from build123d import *

# Parameters (mm, degrees)
SKETCH1_W           = 57.912
SKETCH1_H           = 70.104
SKETCH1_R           = 4.25
SKETCH1_R_2         = 6.35
BOSS_EXTRUDE1_DEPTH = 1.5494
FILLET1_R           = 7.62


with BuildPart() as part:
    # Sketch1 → Boss-Extrude1 (new body)
    with BuildSketch(Plane(origin=(0, 0, 0), x_dir=(0, 0, -1), z_dir=(1, 0, 0))):
        Rectangle(SKETCH1_W, SKETCH1_H)
        with Locations((-20.447, 26.543)):
            Circle(SKETCH1_R, mode=Mode.SUBTRACT)
        with Locations((20.447, 26.543)):
            Circle(SKETCH1_R, mode=Mode.SUBTRACT)
        with Locations((20.447, -26.543)):
            Circle(SKETCH1_R, mode=Mode.SUBTRACT)
        with Locations((-20.447, -26.543)):
            Circle(SKETCH1_R, mode=Mode.SUBTRACT)
        Circle(SKETCH1_R_2, mode=Mode.SUBTRACT)
    extrude(amount=BOSS_EXTRUDE1_DEPTH)

    # Fillet1
    fillet1_edges = [part.edges().sort_by_distance(p)[0] for p in [
        (0.7747, -35.052, -28.956),
        (0.7747, -35.052, 28.956),
        (0.7747, 35.052, 28.956),
        (0.7747, 35.052, -28.956),
    ]]
    fillet(fillet1_edges, radius=FILLET1_R)


solid = part.part
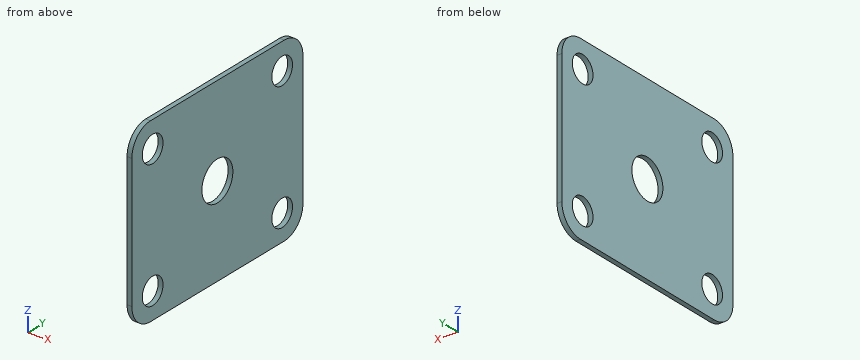
The model under review builds one solid part; all positions refer to its coordinate system, in mm. Give positions to 0.01 mm unless a question says otherwise; leave off trailing zeros. Loops run counter-clockwise (first coordinate to the right, second up) from the corner with the lowest first, then second, coordinate; pieces in that order, holes last. Notation, with made-up numbers: (75.25, 72) -> (131.25, 72) arc R29 cw to (131.25, 102) -> close; hole circle Ø5 at (29, 6.5). An arc over 180 degrees is marked (long way). Write each question's results on one line, items separated by ' | '.
1) Take a section at D-D, the plane z = -22.5. Give the boundary of the cut face in (x, y).
Conclusion:
outline: (0, -34.96) -> (1.55, -34.96) -> (1.55, -30.26) -> (0, -30.26) -> close; (0, -22.82) -> (1.55, -22.82) -> (1.55, 22.82) -> (0, 22.82) -> close; (0, 30.26) -> (1.55, 30.26) -> (1.55, 34.96) -> (0, 34.96) -> close
2) Take a section at C-C, the plane x = 0.75. Give the boundary of the cut face in (y, z), plus the area to 3 significant figures.
Conclusion:
outline: (-35.05, -21.34) arc R7.62 ccw to (-27.43, -28.96) -> (27.43, -28.96) arc R7.62 ccw to (35.05, -21.34) -> (35.05, 21.34) arc R7.62 ccw to (27.43, 28.96) -> (-27.43, 28.96) arc R7.62 ccw to (-35.05, 21.34) -> close; hole circle Ø8.5 at (-26.54, -20.45); hole circle Ø8.5 at (-26.54, 20.45); hole circle Ø12.7 at (0, 0); hole circle Ø8.5 at (26.54, -20.45); hole circle Ø8.5 at (26.54, 20.45) | area: 3,660 mm^2
3) Take a section at B-B, the plane y = 0. Give the boundary of the cut face in (x, z).
Conclusion:
outline: (0, -28.96) -> (1.55, -28.96) -> (1.55, -6.35) -> (0, -6.35) -> close; (0, 6.35) -> (1.55, 6.35) -> (1.55, 28.96) -> (0, 28.96) -> close
4) For line 1 along Z through (x, y) = (0.4, 26.5); line 2 along Y through (x, z) = (0.5, 0); line 3 along Z through (x, y) = (0.75, -28), list the stretches that pass through material, from the lowest coordinate up. Write a range as from..to.
Conclusion:
line 1: z = -28.96..-24.7, -16.2..16.2, 24.7..28.96 | line 2: y = -35.05..-6.35, 6.35..35.05 | line 3: z = -28.93..-24.44, -16.45..16.45, 24.44..28.93
5) Take a section at A-A, the plane z = 0. Give the boundary of the cut face in (x, y), plus the area to 3 significant figures.
Conclusion:
outline: (0, -35.05) -> (1.55, -35.05) -> (1.55, -6.35) -> (0, -6.35) -> close; (0, 6.35) -> (1.55, 6.35) -> (1.55, 35.05) -> (0, 35.05) -> close | area: 88.9 mm^2
6) Insertion check: pin 1 Ø5 at (y, z) = (26.543, 20.447) entering from +X; pin 2 Ø13.5 at (y, z) = (-26.543, 20.447) entering from -X. Each pin has a flat end and moves straight along its axis. Give the tip position at first contact, or say it passes through.
Conclusion:
pin 1: passes through | pin 2: stops at x = 0
